Could you check a few things on this model? Use its own coordinates, in mm. Face numbers are marked on the shaded views. A direction names the side the tool comes from. Coordinates: 2 decimals unless noted, no trailing zeros. Write each loop counter-clockwise with the first axis right and the second up, starting at its lowest first coordinate (ties: lowest second). Pieces come first, ordered by that corner, then holes. Notation, with made-up numbers: (-22, -33.75) - (-2, -33.75) arc R25 cw to (-2, -16.75) - close; hole circle Ø5 at (34, 67). An arc over 180 degrees is marked (long way). Answer as a JSON object with one key per item and string values. Group by question number.
1) If we section it at A-A (z = 4.5): Write out the boundary of the cut face in (x, y), plus the area to 3 significant figures.
2) We'd pull the mould along X, two halves only. Please class the marked faces 4, 5, 6 and 7: released by +X, released by -X, zero draft, split by the parting line, or undercut.
3) On a 3-axis mill with a long thin cutter (end or side, diameter ignored), from which of +Z, -Z, +X, -X, +Y, -Y can I reach the whole of each face in a straight line? I mean the marked faces 1, 2 and 3. Say none if no direction works.
4) If we section it at B-B (x = 0): Write out the boundary of the cut face in (y, z), plus the area to 3 significant figures.
5) Please list where these lines run through material, in increasing order: line 1 along Z through (x, y) = (6, -2); line 2 along X through (y, z) = (0.5, 3.5); line 3 along X through (y, z) = (0, 1).
6) Will these pins go through, and if not, where does the flat tip stop? pin 1 Ø4 at (y, z) = (3.5, 1) entering from -X; pin 2 Ø1.4 at (y, z) = (3.5, 2) entering from +X; pin 3 Ø3.5 at (x, y) = (0, 0) entering from -Z; pin 4 Ø1 at (x, z) = (-2.5, 4.5) entering from -Y.
```python
from build123d import *

# Parameters (mm, degrees)
SKETCH_R        = 1.5
PAD_DEPTH       = 7
SKETCH001_R     = 12
SKETCH001_R_2   = 1.5
PAD001_DEPTH    = 2
CHAMFER_SIZE    = 1
CHAMFER001_SIZE = 1.7


with BuildPart() as part:
    # Sketch → Pad (new body)
    with BuildSketch(Plane.XY):
        with BuildLine():
            ThreePointArc((-2.5, 3.122499), (-3.518971, 1.901799), (-3.981855, 0.380567))
            Line((-5.478695, -0.483634), (-3.981855, 0.380567))
            ThreePointArc((-5.478695, -0.483634), (-4.659167, -2.922699), (-2.81991, -4.722087))
            Line((-1.232265, -3.80546), (-2.81991, -4.722087))
            ThreePointArc((-1.232265, -3.80546), (0.117848, -3.998264), (1.454262, -3.726275))
            Line((2.992718, -4.614503), (1.454262, -3.726275))
            ThreePointArc((2.992718, -4.614503), (4.763149, -2.749985), (5.492638, -0.284484))
            Line((3.954108, 0.604177), (5.492638, -0.284484))
            ThreePointArc((3.954108, 0.604177), (3.46401, 2.000159), (2.5, 3.122499))
            Line((2.5, 3.122499), (2.5, 4.898979))
            ThreePointArc((2.5, 4.898979), (0, 5.5), (-2.5, 4.898979))
            Line((-2.5, 3.122499), (-2.5, 4.898979))
        make_face()
        Circle(SKETCH_R, mode=Mode.SUBTRACT)
    extrude(amount=PAD_DEPTH)

    # Sketch001 (on Face14 of Pad) → Pad001 (join)
    with BuildSketch(Plane(origin=(0, 0, 0), x_dir=(1, 0, 0), z_dir=(0, 0, -1))):
        Circle(SKETCH001_R)
        Circle(SKETCH001_R_2, mode=Mode.SUBTRACT)
    extrude(amount=PAD001_DEPTH)

    # Chamfer
    chamfer_edges = [part.edges().sort_by_distance(p)[0] for p in [
        (-2.026088, -4.263773, 7),
        (0.117848, -3.998264, 7),
        (2.22349, -4.170389, 7),
        (4.763149, -2.749985, 7),
        (3.46401, 2.000159, 7),
        (4.723373, 0.159847, 7),
        (2.5, 4.010739, 7),
        (0, 5.5, 7),
        (-2.5, 4.010739, 7),
        (-3.518971, 1.901799, 7),
        (-4.730275, -0.051534, 7),
        (-4.659167, -2.922699, 7),
    ]]
    chamfer(chamfer_edges, length=CHAMFER_SIZE)

    # Chamfer001
    chamfer001_edges = [part.edges().sort_by_distance(p)[0] for p in [
        (-12, 0, -2),
    ]]
    chamfer(chamfer001_edges, length=CHAMFER001_SIZE)


solid = part.part
```
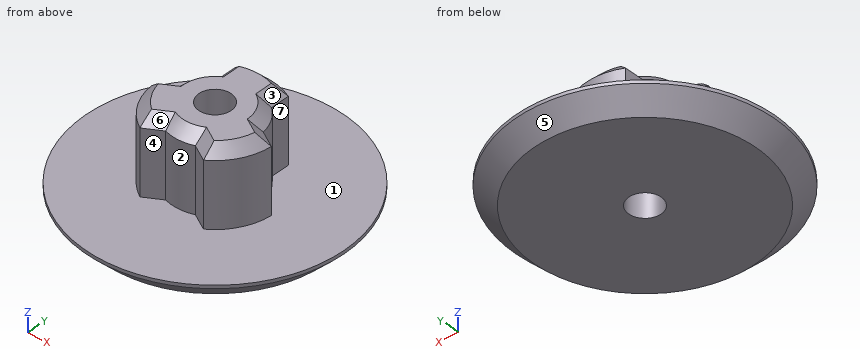
Here are the results:
{
 "1": {"outline": "(-5.48, -0.48) arc R5.5 ccw to (-2.82, -4.72) - (-1.23, -3.81) arc R4 ccw to (1.45, -3.73) - (2.99, -4.61) arc R5.5 ccw to (5.49, -0.28) - (3.95, 0.6) arc R4 ccw to (2.5, 3.12) - (2.5, 4.9) arc R5.5 ccw to (-2.5, 4.9) - (-2.5, 3.12) arc R4 ccw to (-3.98, 0.38) - close; hole circle Ø3 at (0, 0)", "area": "66.9 mm²"},
 "2": {"face 4": "undercut", "face 5": "split by the parting line", "face 6": "undercut", "face 7": "released by +X"},
 "3": {"face 1": "+Z", "face 2": "+Z, -Y", "face 3": "+Z, +X, +Y"},
 "4": {"outline": "(-12, -0.3) - (-10.3, -2) - (-1.5, -2) - (-1.5, 7) - (-3, 7) - (-4, 6) - (-4, 0) - (-12, 0) - close; (1.5, -2) - (10.3, -2) - (12, -0.3) - (12, 0) - (5.5, 0) - (5.5, 6) - (4.5, 7) - (1.5, 7) - close", "area": "83.6 mm²"},
 "5": {"line 1": "z = -2 to 0", "line 2": "x = -3.97 to -1.41, 1.41 to 4.13", "line 3": "x = -4.64 to -1.5, 1.5 to 5"},
 "6": {"pin 1": "stops at x = -11.87", "pin 2": "stops at x = 2.86", "pin 3": "stops at z = -2", "pin 4": "stops at y = -4.72"}
}
